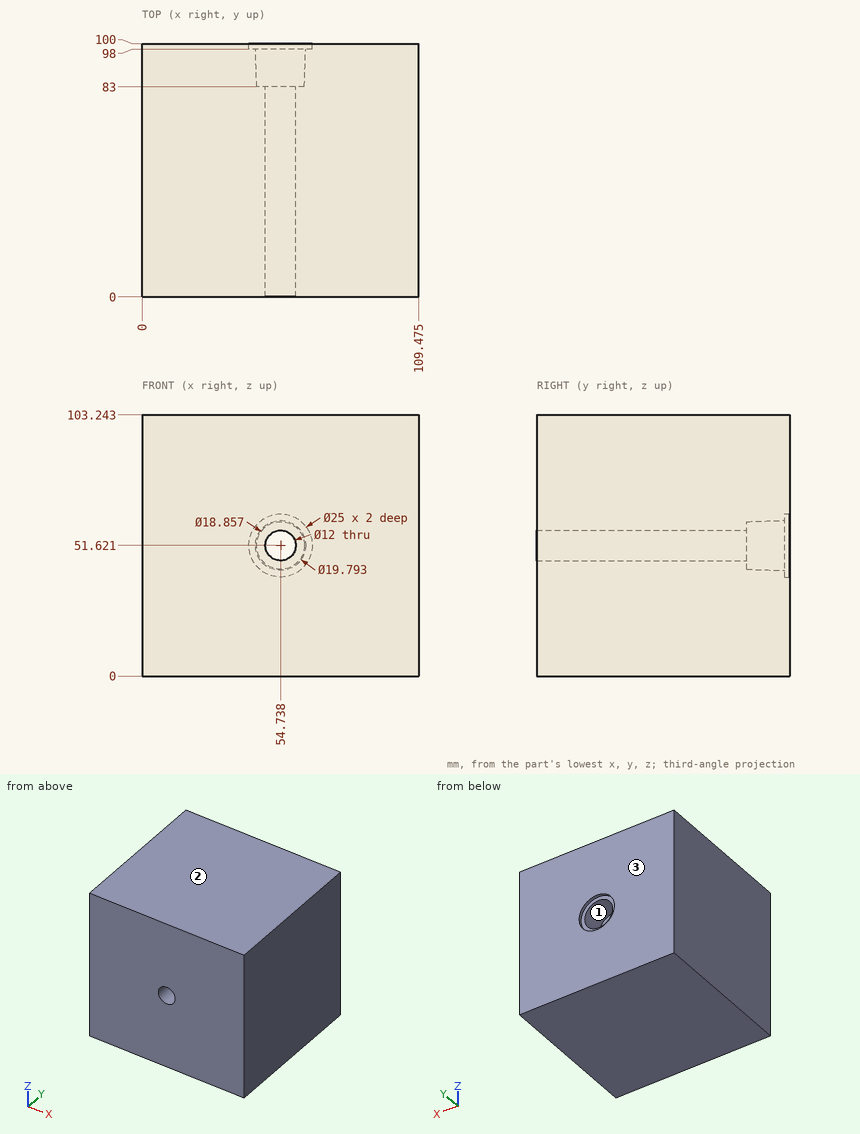
Study the drawing (mm; zero at the part's minimum x, y, z) and answer. Coordinates: 2 decimals unless noted, no trailing zeros. Write each question's results on one line, items separated by ' | '.
Item 1: For a pull along Z with two mould halves and no side action, classify the marked faces 1, 2 and 3 as released by +Z, released by -Z, zero draft, split by the parting line, or undercut.
Answer below:
face 1: undercut | face 2: released by +Z | face 3: zero draft
Item 2: Consider probe 1 along X at (y, z) = (26, 51) (1 decimal); probe 2 along Z at (x, y) = (50, 80.5) (1 decimal); probe 3 along Y at (x, z) = (45, 54.5). Determine where each line is inside the solid, lowest interval first. Write a range as [from, to].
Answer below:
probe 1: [0, 48.8], [60.7, 109.5] | probe 2: [0, 47.9], [55.3, 103.2] | probe 3: [0, 98]
Item 3: Given P1, Ø7.5, axis at x = 59.5, z = 57.5, coming from the +Y side; P2, Ø15, axis at x = 53.5, z = 50.5, coming from the +Y side, each flat-ended and moving along its own axis, determine where each tip first touches the part or whether it passes through.
Answer below:
P1: y = 98 | P2: y = 83
